```python
from build123d import *

# Parameters (mm, degrees)
SKETCH_1_W      = 110
SKETCH_1_H      = 35
EXTRUDE_1_DEPTH = 13.5
REVOLVE_1_ANGLE = 90


with BuildPart() as part:
    # 草圖1 → 填料-伸長1 (new body, symmetric)
    with BuildSketch(Plane.XY):
        Rectangle(SKETCH_1_W, SKETCH_1_H)
    extrude(amount=EXTRUDE_1_DEPTH, both=True)

    # 草圖2 → 旋轉1 (revolve)
    with BuildSketch(Plane.ZY.offset(55)):
        with BuildLine():
            Line((-2.5, -12.5), (2.5, -12.5))
            ThreePointArc((2.5, -12.5), (5, -15), (2.5, -17.5))
            Line((2.5, -17.5), (-2.5, -17.5))
            ThreePointArc((-2.5, -17.5), (-5, -15), (-2.5, -12.5))
        make_face()
    revolve(axis=Axis((-55, -24.005362061, -6.079544695), (0, 0, 1)), revolution_arc=REVOLVE_1_ANGLE)


solid = part.part
```
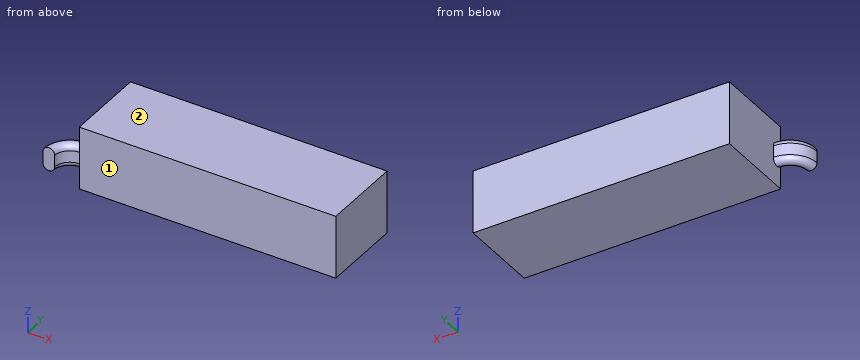
Geometry check sheet. Reference: the model listing, model coordinates, mm. Face numbers are marked on the shaded views. A direction names the side the tool comes from. Round coordinates to 2 decimals unless told otherwise and drop trailing zeros. Write each loop counter-clockwise with the first axis right and the second up, starting at its lowest first coordinate (ties: lowest second). Pieces come first, ordered by that corner, then holes. Notation, with made-up numbers: (1.25, -13) - (46.25, -13) arc R13 cw to (46.25, 12) - close; hole circle Ø3 at (32, -36). An arc over 180 degrees is marked (long way). Write each question's results on one line, items separated by ' | '.
(1) Sectioned sample at A-A, the plane x = -15.5. Enter the section's corners in (y, z).
Computed:
outline: (-17.5, -13.5) - (17.5, -13.5) - (17.5, 13.5) - (-17.5, 13.5) - close
(2) Depth check by flat-ended pin: pin 1 Ø10 at (y, z) = (-12.5, 5.5) entering from -X; pin 2 Ø2 at (x, z) = (1.5, 1) entering from -Y; pin 3 Ø10 at (y, z) = (5.5, -4) entering from -X. Enter the tip coordinate at first touch or a pass-through.
Computed:
pin 1: stops at x = -63.95 | pin 2: stops at y = -17.5 | pin 3: stops at x = -55
(3) Thickness scan on probe 1 along Y at (x, z) = (4.5, 4.75); probe 2 along X at (y, z) = (-6.5, -9.5); probe 3 along X at (y, z) = (-20.5, -1.75). Record the ranges inside material, lowest first. Write a range as from..to.
Computed:
probe 1: y = -17.5..17.5 | probe 2: x = -55..55 | probe 3: x = -65.96..-60.48
(4) Sectioned sample at B-B, the plane z = 9.5. Enter the section's corners in (x, y), plus the area to 3 significant figures.
Computed:
outline: (-55, -17.5) - (55, -17.5) - (55, 17.5) - (-55, 17.5) - close | area: 3,850 mm^2
(5) Set-up check for the marked faces 1 and 2: record each of +Z, -Z, +X, -X, +Y, -Y from which the full face is reachable in a straight line by a thin tool's end or side.
Computed:
face 1: +Z, -Z, +X, -Y | face 2: +Z, +X, -X, +Y, -Y
